CAD build for the part. Positions are in the model's coordinates, mm. Face numbers are marked on the shaded views. A direction names the side the tool comes from. Coordinates: 2 decimals unless noted, no trailing zeros. Write each loop counter-clockwise with the first axis right and the second up, starting at its lowest first coordinate (ties: lowest second). Pieces come first, ordered by that corner, then holes.
```python
from build123d import *

# Parameters (mm, degrees)
F0_R      = 17
F1_DEPTH  = 4
F2_R      = 12.5
F3_DEPTH  = 1
F4_R      = 5
F5_DEPTH  = 1
F6_R      = 2.5
F7_DEPTH  = 1
F8_R      = 2.848441
F9_DEPTH  = 5
F10_R     = 0.607579
F11_DEPTH = 0.5
F12_R     = 3
F13_DEPTH = 9
F14_R     = 2.131579
F15_DEPTH = 8


with BuildPart() as f1:
    # F0 (on Front) → F1 (new body)
    with BuildSketch(Plane.XZ):
        Circle(F0_R)
    extrude(amount=F1_DEPTH)

    # F2 (on face) → F3 (cut)
    with BuildSketch(Plane.XZ.offset(4)):
        Circle(F2_R)
    extrude(amount=-F3_DEPTH, mode=Mode.SUBTRACT)

    # F4 (on face) → F5 (join)
    with BuildSketch(Plane.XZ.offset(3)):
        Circle(F4_R)
    extrude(amount=F5_DEPTH)

    # F6 (on face) → F7 (join)
    with BuildSketch(Plane.XZ.offset(4)):
        Circle(F6_R)
    extrude(amount=F7_DEPTH)

    # F8 (on face) → F9 (cut)
    with BuildSketch(Plane.XZ.offset(3)):
        with Locations((-6.152258, 6.152258)):
            Circle(F8_R)
        with Locations((-8.700607, 0)):
            Circle(F8_R)
        with Locations((-6.152258, -6.152258)):
            Circle(F8_R)
        with Locations((0, -8.700607)):
            Circle(F8_R)
        with Locations((6.152258, -6.152258)):
            Circle(F8_R)
        with Locations((8.700607, 0)):
            Circle(F8_R)
        with Locations((6.152258, 6.152258)):
            Circle(F8_R)
        with Locations((0, 8.700607)):
            Circle(F8_R)
    extrude(amount=-F9_DEPTH, mode=Mode.SUBTRACT)

    # F10 (on face) → F11 (join)
    with BuildSketch(Plane.XZ.offset(4)):
        with Locations((0, 3.731649)):
            Circle(F10_R)
        with Locations((-2.193408, 3.018968)):
            Circle(F10_R)
        with Locations((-3.549009, 1.153143)):
            Circle(F10_R)
        with Locations((-3.549009, -1.153143)):
            Circle(F10_R)
        with Locations((-2.193408, -3.018968)):
            Circle(F10_R)
        with Locations((0, -3.731649)):
            Circle(F10_R)
        with Locations((2.193408, -3.018968)):
            Circle(F10_R)
        with Locations((3.549009, -1.153143)):
            Circle(F10_R)
        with Locations((3.549009, 1.153143)):
            Circle(F10_R)
        with Locations((2.193408, 3.018968)):
            Circle(F10_R)
    extrude(amount=F11_DEPTH)

    # F12 (on face) → F13 (join)
    with BuildSketch(Plane(origin=(0, 0, 0), x_dir=(-1, 0, 0), z_dir=(0, 1, 0))):
        Circle(F12_R)
    extrude(amount=F13_DEPTH)

    # F14 (on face) → F15 (cut)
    with BuildSketch(Plane(origin=(0, 9, 0), x_dir=(-1, 0, 0), z_dir=(0, 1, 0))):
        Circle(F14_R)
    extrude(amount=-F15_DEPTH, mode=Mode.SUBTRACT)


solid = f1.part
```
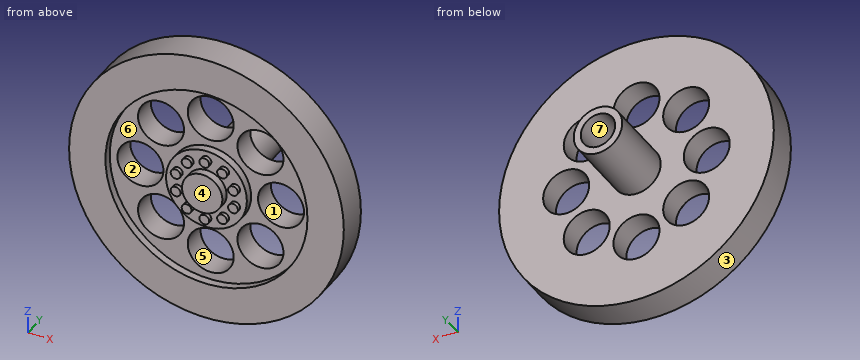
Item 1: Two-plate mould, pull along Z, no slides. Class the marked faces 1, 2, 3 and 4: +Z half, -Z half, draft (parallel to the pull), parting line (faces both ways), or undercut.
Item 2: Saw through at A-A, the plane z = 0. State how many separate pieces and enclosed holes the cut face has, and give its area (3 significant figures).
Item 3: Saw through at C-C, the plane z = -11. Write the cut outline in (x, y), and give its area (3 significant figures).
Item 4: Which spindle directions (+Z, -Z, +X, -X, +Y, -Y) get a long thin tool onto all of the face, cutting with end or side? Do the marked faces 5, 6 and 7. Say none if no direction does.
Item 5: Flat gauge pins, fed straight in: pin 1 Ø3 at (y, z) = (-3.5, 9) entering from -X; pin 2 Ø2 at (x, z) = (-6.5, 12.5) entering from +Y; pin 3 Ø5 at (x, z) = (10.5, 13.5) entering from -Y; pin 4 Ø4 at (x, y) = (6.5, 4.5) entering from +Z. Where does each tip first touch, or does it go through?
Item 6: Saw through at B-B, the plane x = -7. Write the cut outline in (y, z).
Item 7: Wall check: line 1 along X through (y, z) = (-1, 5); line 2 along Z through (x, y) = (4.5, -1.75); line 3 along Y through (x, z) = (0, 1.5). Give the ranges that are in metal, low to high.
Working result:
1. face 1: undercut
1. face 2: undercut
1. face 3: parting line
1. face 4: draft
2. separate pieces: 3
2. enclosed holes: 0
2. area: 112 mm2
3. outline: (-12.96, -4) - (-5.94, -4) - (-5.94, -3) - (-1.68, -3) - (-1.68, 0) - (-12.96, 0) - close; (1.68, -3) - (5.94, -3) - (5.94, -4) - (12.96, -4) - (12.96, 0) - (1.68, 0) - close
3. area: 81.7 mm2
4. face 5: +Y, -Y
4. face 6: -Y
4. face 7: +Y
5. pin 1: stops at x = -15.26
5. pin 2: stops at y = 0
5. pin 3: stops at y = -4
5. pin 4: passes through
6. outline: (-4, -15.49) - (0, -15.49) - (0, -8.87) - (-3, -8.87) - (-3, -10.36) - (-4, -10.36) - close; (-4, 10.36) - (-3, 10.36) - (-3, 8.87) - (0, 8.87) - (0, 15.49) - (-4, 15.49) - close; (-3, -3.43) - (0, -3.43) - (0, -2.29) - (-3, -2.29) - close; (-3, 2.29) - (0, 2.29) - (0, 3.43) - (-3, 3.43) - close
7. line 1: x = -16.25 to -8.76, -3.55 to 3.55, 8.76 to 16.25
7. line 2: z = -16.39 to -8.47, -3.83 to 3.83, 8.47 to 16.39
7. line 3: y = -5 to 1
